The figure shows three views and two pictorial views of one solid part (mm, origin at its lowest corner). Answer the questions. A direction names the side the tool comes from. Coordinates: 2 decimals unless noted, no trailing zeros. Loops run counter-clockwise (first coordinate to the right, second up) from the corner with the lowest first, then second, coordinate; pieces in that order, holes last.
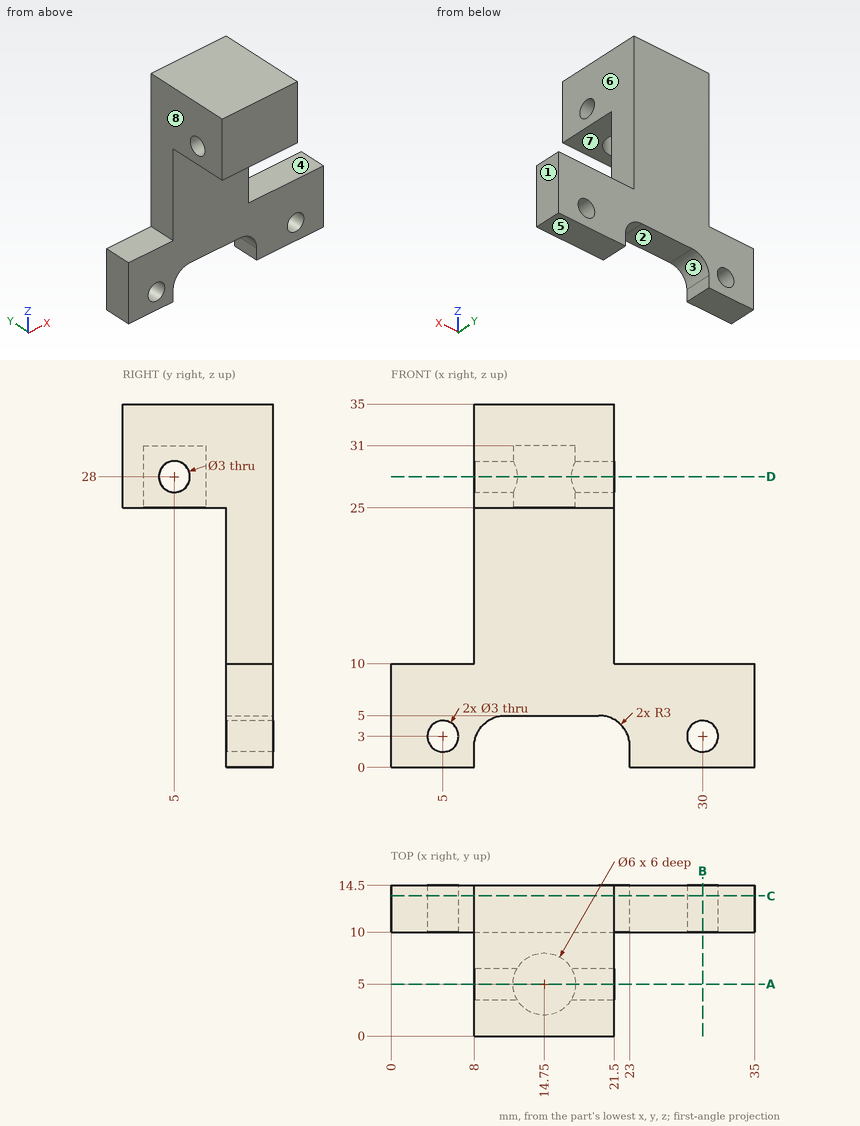
Q1. Flat-ended cylindrical pins translate along their axes: pin 1 Ø2.5 at (y, z) = (5, 28) entering from +X; pin 2 Ø8 at (x, y) = (14.75, 5) entering from -Z; pin 3 Ø6 at (y, z) = (13, 14.5) entering from -X; pin 4 Ø1.8 at (x, y) = (15, 6.5) entering from -Z. Find the tip coordinate at first contact, or state that the pin passes through.
Findings below:
pin 1: passes through
pin 2: stops at z = 25
pin 3: stops at x = 8
pin 4: stops at z = 31
Q2. Which of the six approach directions +Z, -Z, +X, -X, +Y, -Y give full straight-line access (tool end or side, diameter ignored) to the marked faces 5, 6, 7 and 8?
Findings below:
face 5: -Z, +X, -X, +Y, -Y
face 6: +Z, +X, +Y, -Y
face 7: -Z, +X, -X, -Y
face 8: +Z, -X, +Y, -Y
Q3. Determine the mould class of the marked faces 1, 2, 3 and 4 for opening direction X: +X half, -X half, draft (parallel to the pull), parting line (faces both ways), or undercut.
Findings below:
face 1: +X half
face 2: undercut
face 3: undercut
face 4: draft
Q4. A cutting plane is placed at A-A (y = 5). Give the vertices of the cut face in (x, z), then the cut area to 3 significant figures.
Findings below:
outline: (8, 25) - (11.75, 25) - (11.75, 26.5) - (8, 26.5) - close; (8, 29.5) - (11.75, 29.5) - (11.75, 31) - (17.75, 31) - (17.75, 29.5) - (21.5, 29.5) - (21.5, 35) - (8, 35) - close; (17.75, 25) - (21.5, 25) - (21.5, 26.5) - (17.75, 26.5) - close
area: 76.5 mm2
Q5. Straight lines are drawn through the part: probe 1 along Z at (x, y) = (5, 13.25); probe 2 along Y at (x, z) = (10.35, 28); probe 3 along Y at (x, z) = (14.75, 27). For each, find the intervals that lie inside material, in ascending order.
Findings below:
probe 1: z = 0 to 1.5, 4.5 to 10
probe 2: y = 0 to 3.5, 6.5 to 14.5
probe 3: y = 0 to 2, 8 to 14.5
Q6. A cutting plane is placed at C-C (y = 13.5). Give the vertices of the cut face in (x, z).
Findings below:
outline: (0, 0) - (8, 0) - (8, 2) arc R3 cw to (11, 5) - (20, 5) arc R3 cw to (23, 2) - (23, 0) - (35, 0) - (35, 10) - (21.5, 10) - (21.5, 35) - (8, 35) - (8, 10) - (0, 10) - close; hole circle Ø3 at (5, 3); hole circle Ø3 at (30, 3)
Q7. A cutting plane is placed at D-D (z = 28). Give the vertices of the cut face in (x, y), then the cut area to 3 significant figures.
Findings below:
outline: (8, 0) - (21.5, 0) - (21.5, 3.5) - (17.35, 3.5) arc R3 cw to (12.15, 3.5) - (8, 3.5) - close; (8, 6.5) - (12.15, 6.5) arc R3 cw to (17.35, 6.5) - (21.5, 6.5) - (21.5, 14.5) - (8, 14.5) - close
area: 144 mm2
Q8. A cutting plane is placed at B-B (x = 30). Give the vertices of the cut face in (y, z), then the cut area to 3 significant figures.
Findings below:
outline: (10, 0) - (14.5, 0) - (14.5, 1.5) - (10, 1.5) - close; (10, 4.5) - (14.5, 4.5) - (14.5, 10) - (10, 10) - close
area: 31.5 mm2
